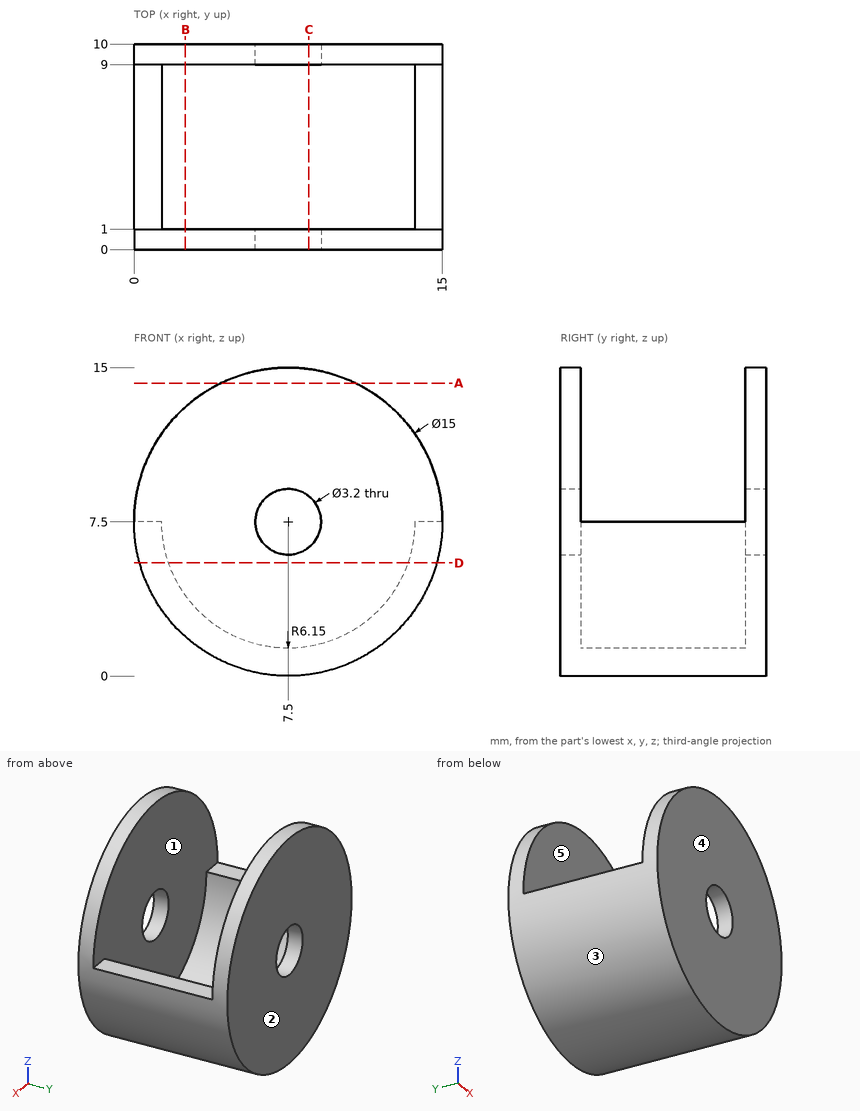
Part print with two shaded views. Sizes in mm from the minimum x, y, z corner. A direction names the side the tool comes from. Coordinates: 2 decimals unless noted, no trailing zeros. Order: outer loops, then holes, each group sorted by start corner. A loop starts at its lowest first (then second) coordinate and runs counter-clockwise, first axis right, second up.
(1) Pin check, flat tips, straight feed: pin 1 Ø1.5 at (x, y) = (14.5, 3.5) entering from +Z; pin 2 Ø3 at (x, z) = (7.5, 7.5) entering from -Y; pin 3 Ø1 at (y, z) = (8.5, 2.5) entering from +X; pin 4 Ø2 at (y, z) = (4.5, 6) entering from +X. Stop position of each tip, or through.
Solution:
pin 1: stops at z = 7.5
pin 2: passes through
pin 3: stops at x = 13.5
pin 4: stops at x = 14.98
(2) Saw through at B-B, the plane x = 2.5. Write the cut outline in (y, z), and give its area (3 significant figures).
Solution:
outline: (0, 1.91) - (10, 1.91) - (10, 13.09) - (9, 13.09) - (9, 3.92) - (1, 3.92) - (1, 13.09) - (0, 13.09) - close
area: 38.4 mm2
(3) Saw through at C-C, the plane x = 8.5. Write the cut outline in (y, z).
Solution:
outline: (0, 0.07) - (10, 0.07) - (10, 6.25) - (9, 6.25) - (9, 1.43) - (1, 1.43) - (1, 6.25) - (0, 6.25) - close; (0, 8.75) - (1, 8.75) - (1, 14.93) - (0, 14.93) - close; (9, 8.75) - (10, 8.75) - (10, 14.93) - (9, 14.93) - close
(4) Mould opens along X. For the marked faces 1, 2 and 3 say: released by +X, released by -X, zero draft, split by the parting line, or undercut.
Solution:
face 1: undercut
face 2: zero draft
face 3: split by the parting line
(5) Saw through at D-D, the plane z = 5.5. Write the cut outline in (x, y).
Solution:
outline: (0.27, 0) - (14.73, 0) - (14.73, 10) - (0.27, 10) - close; hole (1.68, 1) - (13.32, 1) - (13.32, 9) - (1.68, 9) - close
(6) Drill centre lines: L1, parallel to Z at x = 7.5, y = 0.55; L2, parallel to Y at x = 9.5, z = 4.5. Where is each one in solid material? Low to high.
Solution:
L1: z = 0 to 5.9, 9.1 to 15
L2: y = 0 to 1, 9 to 10
(7) Which spindle directions (+Z, -Z, +X, -X, +Y, -Y) get a long thin tool onto all of the face, cutting with end or side? Do the marked faces 4 and 5. Say none if no direction does.
Solution:
face 4: +Z, -Z, +X, -X, -Y
face 5: +Z
(8) Saw through at A-A, the plane z = 14.25. Write the cut outline in (x, y).
Solution:
outline: (4.23, 0) - (10.77, 0) - (10.77, 1) - (4.23, 1) - close; (4.23, 9) - (10.77, 9) - (10.77, 10) - (4.23, 10) - close
